Can you work these out from the model? Positions are in its coordinate system, mm. Round coordinates to 2 decimals unless told otherwise and drop trailing zeros. Loops run counter-clockwise (first coordinate to the right, second up) from the corner with the lowest first, then second, coordinate; pieces in that order, holes last.
Autodesk Inventor part; units mm, degrees
ref_plane "YZ Plane" through (0, 0, 0) normal (1, 0, 0) x (0, 1, 0)
ref_plane "XZ Plane" through (0, 0, 0) normal (0, 1, 0) x (-1, 0, 0)
ref_plane "XY Plane" through (0, 0, 0) normal (0, 0, 1) x (1, 0, 0)
sketch "Эскиз1" plane through (0, 0, 0) normal (0, 1, 0) x (-1, 0, 0)
  line L0 (-80, 144) -> (80, 144)
  line L1 (80, 144) -> (80, -144)
  line L2 (80, -144) -> (-80, -144)
  line L3 (-80, -144) -> (-80, 144)
  line L4 (-80, 144) -> (80, -144) construction
  line L5 (80, 144) -> (-80, -144) construction
  point P0 (0, 0)
  dimension "d0" = 160
  dimension "d1" = 288
extrude "Выдавливание1" add sketch "Эскиз1" along normal blind 6
sketch "Эскиз4" plane through (0, 6, 0) normal (0, 1, 0) x (1, 0, 0)
  circle A0 centre (63.6396, 63.6396) radius 4
  line L0 (0, 0) -> (31.2937, 0) construction
  line L1 (63.6396, 63.6396) -> (0, 0) construction
  dimension "d8" = 8
  dimension "d9" = 90
  dimension "d10" = 45
extrude "Выдавливание4" [suppressed]
pattern_circular "Круговой массив1" [suppressed]
sketch "Эскиз6" plane through (0, 0, 0) normal (0, -1, 0) x (1, 0, 0)
  circle A0 centre (-61.2673, 61.2541) radius 4
  circle A1 centre (-61.2673, -61.2603) radius 4
  circle A2 centre (61.2471, -61.2603) radius 4
  circle A3 centre (61.2471, 61.2541) radius 4
  circle A4 centre (20.3596, -84) radius 26.5
  circle A5 centre (20.3596, 84) radius 26.5
  point P0 (0, 0)
extrude "Выдавливание5" cut sketch "Эскиз6" against normal blind 10
sketch "Эскиз7" plane through (0, 0, 0) normal (0, -1, 0) x (1, 0, 0)
  circle A0 centre (-13.5545, -70.7681) radius 1.5
  circle A1 centre (54.2737, -97.2319) radius 1.5
  circle A2 centre (54.2737, 97.2319) radius 1.5
  circle A3 centre (-13.5545, 70.7681) radius 1.5
  point P0 (0, 0)
extrude "Выдавливание6" cut sketch "Эскиз7" against normal blind 10
sketch "Эскиз8" plane through (0, 0, 0) normal (0, -1, 0) x (1, 0, 0)
  circle A0 centre (-68.825, -100.977) radius 2
  circle A1 centre (-68.825, -88.977) radius 2
  circle A2 centre (-53.825, -90.977) radius 2
  circle A3 centre (-53.825, -108.4524) radius 2
  point P0 (0, 0)
extrude "Выдавливание7" cut sketch "Эскиз8" against normal blind 10
sketch "Эскиз9" plane through (0, 0, 0) normal (0, -1, 0) x (1, 0, 0)
  circle A0 centre (72.875, -128) radius 2
  circle A1 centre (-72.875, -128) radius 2
  circle A2 centre (-72.875, 128) radius 2
  circle A3 centre (72.875, 128) radius 2
  point P0 (0, 0)
sketch "Эскиз10" plane through (0, 0, 0) normal (0, -1, 0) x (1, 0, 0)
  arc A0 (80, -83.696) -> (80, -121.0515) centre (80.1966, -102.3738) ccw
  line L0 (80, 144) -> (80, -144)
  point P0 (0, 0)
extrude "Выдавливание8" cut sketch "Эскиз10" against normal blind 10
sketch "Эскиз11" plane through (0, 0, 0) normal (0, -1, 0) x (1, 0, 0)
  circle A0 centre (-64.4611, 0) radius 4
  line L0 (-80, -144) -> (-80, 144)
  point P0 (0, 0)
  point P1 (-80, 0)
  dimension "d24" = 8
extrude "Выдавливание9" cut sketch "Эскиз11" against normal through all
extrude "Выдавливание10" cut sketch "Эскиз9" against normal through all
properties part number "000.001.006 - Площадка под манипулятор"
(1) If we section it at C-C, the plane z = 0: List the corners of the cut face in (x, y) for me, then the cut area to 3 significant figures.
Worked answers:
outline: (-80, 0) - (-68.46, 0) - (-68.46, 6) - (-80, 6) - close; (-60.46, 0) - (80, 0) - (80, 6) - (-60.46, 6) - close
area: 912 mm2
(2) Will this pin go through, and if not, where does the flat tip stop? P1, Ø1.8, axis at x = 54.27, z = 97.23, coming from the -Y side.
Worked answers:
P1: passes through
(3) If we section it at D-D, the plane z = -117: List the corners of the cut face in (x, y) for me, then the cut area to 3 significant figures.
Worked answers:
outline: (-80, 0) - (68.58, 0) - (68.58, 6) - (-80, 6) - close
area: 891 mm2
(4) If we mould it in two halves opening along X, with no side actions, what happens to faces 1 (the flat face through (80, 3, -133)), 2 (the cylindrical face through (-59.422, 2.958, 57.705)), 3 (the flat face through (1, 6, 2))? For each: released by +X, released by -X, zero draft, split by the parting line, or undercut.
Worked answers:
face 1: released by +X
face 2: undercut
face 3: zero draft
(5) If I drill on line 1 (X direction, y = 3.05, z = 128) (3 decimals); line 2 (Z direction, x = 15, y = 1.75); line 3 (Z direction, x = 10, y = 1.9), over which ranges is the centre line in solid material (lowest first)?
Worked answers:
line 1: x = -80 to -74.875, -70.875 to 70.875, 74.875 to 80
line 2: z = -144 to -109.95, -58.05 to 58.05, 109.95 to 144
line 3: z = -144 to -108.39, -59.61 to 59.61, 108.39 to 144
(6) If we section it at B-B, the plane y = 1.2: State how many separate pieces and enclosed holes the cut face has, then the cut area to 3 significant figures.
Worked answers:
separate pieces: 1
enclosed holes: 19
area: 40,700 mm2
(7) If we section it at A-A, the plane z = 84: List the corners of the cut face in (x, y) for me, then the cut area to 3 significant figures.
Worked answers:
outline: (-80, 0) - (-6.14, 0) - (-6.14, 6) - (-80, 6) - close; (46.86, 0) - (80, 0) - (80, 6) - (46.86, 6) - close
area: 642 mm2
